Source: CAD feature listing. Evaluate the final solid. Frame: model axes, mm. Give positions to 0.01 mm unless a question says otherwise; leave off trailing zeros. Loops run counter-clockwise (first coordinate to the right, second up) from the corner with the lowest first, then second, coordinate; pieces in that order, holes last. Notation, with made-up numbers: (-8.5, -15.5) -> (6.5, -15.5) arc R22 cw to (6.5, -8.5) -> close; hole circle Ø8 at (50.5, 46.25). An arc over 180 degrees is marked (long way). Return JSON: item names as keys, results as strings. Group by question number.
(1) Cut plane A-A on z = 127. Return loops of the section in (x, y).
(2) Ray query, line 1 (X direction, y = 6, z = 74.5); line 2 (Y direction, x = -2.5, z = 513); line 3 (Z direction, x = -15.75, y = 26). Return the intervals inside material, ascending. Write a range as from..to.
(3) Cut plane D-D on z = 530.5. Return loops of the section in (x, y), then the cut area to 3 significant figures.
(4) Cut plane B-B on x = -9.75. Return loops of the section in (y, z).
(5) Cut plane C-C on y = 26. Give the number of separate pieces and of enclosed holes in the cut face, then the cut area to 3 significant figures.
```python
from build123d import *

# Parameters (mm, degrees)
F0_W     = 25.4
F0_H     = 50.8
F1_DEPTH = 609.6
F2_W     = 19.05
F2_H     = 44.45
F3_DEPTH = 670.56
F4_R     = 14.2875
F5_DEPTH = 83.82


with BuildPart() as f1:
    # F0 (on Top) → F1 (new body)
    with BuildSketch(Plane.XY):
        with Locations((-5.123792, 24.444854)):
            Rectangle(F0_W, F0_H)
    extrude(amount=F1_DEPTH)

    # F2 (on face) → F3 (cut)
    with BuildSketch(Plane.XY.offset(609.6)):
        with Locations((-5.123792, 24.444854)):
            Rectangle(F2_W, F2_H)
    extrude(amount=-F3_DEPTH, mode=Mode.SUBTRACT)

    # F4 (on face) → F5 (cut)
    with BuildSketch(Plane.YZ.offset(7.576208)):
        with Locations((24.444854, 304.8)):
            Circle(F4_R)
        with Locations((24.444854, 482.6)):
            Circle(F4_R)
        with Locations((24.444854, 127)):
            Circle(F4_R)
    extrude(amount=-F5_DEPTH, mode=Mode.SUBTRACT)


solid = f1.part
```
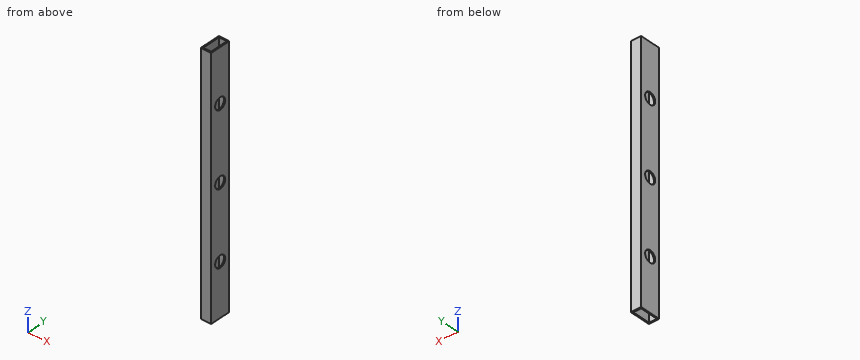
Answers:
{
 "1": {"outline": "(-17.82, -0.96) -> (7.58, -0.96) -> (7.58, 10.16) -> (4.4, 10.16) -> (4.4, 2.22) -> (-14.65, 2.22) -> (-14.65, 10.16) -> (-17.82, 10.16) -> close; (-17.82, 38.73) -> (-14.65, 38.73) -> (-14.65, 46.67) -> (4.4, 46.67) -> (4.4, 38.73) -> (7.58, 38.73) -> (7.58, 49.84) -> (-17.82, 49.84) -> close"},
 "2": {"line 1": "-17.82..-14.65, 4.4..7.58", "line 2": "-0.96..2.22, 46.67..49.84", "line 3": "0..112.8, 141.2..290.6, 319..468.4, 496.8..609.6"},
 "3": {"outline": "(-17.82, -0.96) -> (7.58, -0.96) -> (7.58, 49.84) -> (-17.82, 49.84) -> close; hole (-14.65, 2.22) -> (4.4, 2.22) -> (4.4, 46.67) -> (-14.65, 46.67) -> close", "area": "444 mm²"},
 "4": {"outline": "(-0.96, 0) -> (2.22, 0) -> (2.22, 609.6) -> (-0.96, 609.6) -> close; (46.67, 0) -> (49.84, 0) -> (49.84, 609.6) -> (46.67, 609.6) -> close"},
 "5": {"separate pieces": "8", "enclosed holes": "0", "area": "3,330 mm²"}
}
